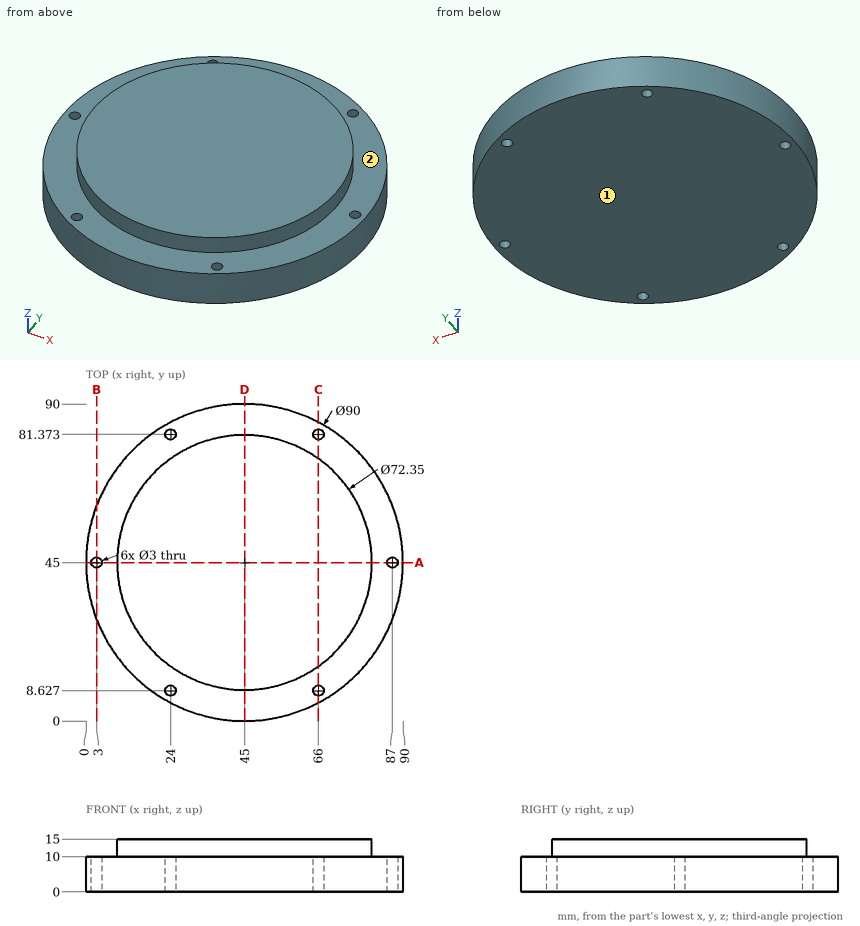
Job drawing, mm, ordinate dimensions from the low corner. One solid piece. A direction names the side the tool comes from. Give positions to 0.01 mm unless a question says otherwise; leave off trailing zeros. Loops run counter-clockwise (first coordinate to the right, second up) from the corner with the lowest first, then second, coordinate; pieces in that order, holes last. Notation, with made-up numbers: (-4.5, -18) -> (23.5, -18) arc R19 cw to (23.5, -4) -> close; hole circle Ø9 at (73.5, 23). An arc over 180 degrees is marked (long way). Use a Markdown table: item, result. Add a question column.
(1) Slice it at D-D on x = 45. List the corners of the cut face in (y, z) (3 decimals).
(2) Slice it at C-C on x = 66. List the corners of the cut face in (y, z), and give its area (3 significant figures).
(3) Wall check: line 1 along Y through (x, z) = (66, 2.75); line 2 along X through (y, z) = (82, 9.5); line 3 along Z through (x, y) = (7, 61). Give the ranges that are in metal, low to high.
(4) Slice it at B-B on x = 3. List the corners of the cut face in (y, z), and give its area (3 significant figures).
(5) Drop flat-ended pins along their axis: pin 1 Ø4 at (x, z) = (25, 11.5) entering from +Y; pin 2 Ø2.5 at (x, y) = (3, 45) entering from -Z; pin 3 Ø6 at (y, z) = (77.5, 11) entering from +X; pin 4 Ø2 at (x, z) = (70.5, 6.5) entering from +Y. Give the stop position or say it passes through.
(6) Tool access for the marked faces 1 and 2: list every direction of +Z, -Z, +X, -X, +Y, -Y with a clear straight run to the whole face (end or side of a thin tool).
(7) Slice it at A-A on y = 45. List the corners of the cut face in (x, z) (3 decimals).
Filled sheet:
| question | item | result |
|---|---|---|
| 1 | outline | (0, 0) -> (90, 0) -> (90, 10) -> (81.175, 10) -> (81.175, 15) -> (8.825, 15) -> (8.825, 10) -> (0, 10) -> close |
| 2 | outline | (5.2, 0) -> (7.13, 0) -> (7.13, 10) -> (5.2, 10) -> close; (10.13, 0) -> (79.87, 0) -> (79.87, 10) -> (74.46, 10) -> (74.46, 15) -> (15.54, 15) -> (15.54, 10) -> (10.13, 10) -> close; (82.87, 0) -> (84.8, 0) -> (84.8, 10) -> (82.87, 10) -> close |
| 2 | area | 1,030 mm2 |
| 3 | line 1 | 5.2 to 7.13, 10.13 to 79.87, 82.87 to 84.8 |
| 3 | line 2 | 19.39 to 22.64, 25.36 to 64.64, 67.36 to 70.61 |
| 3 | line 3 | 0 to 10 |
| 4 | outline | (28.84, 0) -> (43.5, 0) -> (43.5, 10) -> (28.84, 10) -> close; (46.5, 0) -> (61.16, 0) -> (61.16, 10) -> (46.5, 10) -> close |
| 4 | area | 293 mm2 |
| 5 | pin 1 | y = 85.94 |
| 5 | pin 2 | through |
| 5 | pin 3 | x = 78.83 |
| 5 | pin 4 | y = 82.75 |
| 6 | face 1 | -Z, +X, -X, +Y, -Y |
| 6 | face 2 | +Z |
| 7 | outline | (0, 0) -> (1.5, 0) -> (1.5, 10) -> (0, 10) -> close; (4.5, 0) -> (85.5, 0) -> (85.5, 10) -> (81.175, 10) -> (81.175, 15) -> (8.825, 15) -> (8.825, 10) -> (4.5, 10) -> close; (88.5, 0) -> (90, 0) -> (90, 10) -> (88.5, 10) -> close |
